Part model, mm, in its own coordinate system. A direction names the side the tool comes from. Give positions to 0.01 mm unless a question says otherwise; leave off trailing zeros. Write each loop counter-clockwise with the first axis right and the second up, starting at its lowest first coordinate (ties: lowest second). Pieces come first, ordered by that corner, then holes. Notation, with made-up numbers: (5, 84.25) - (45, 84.25) arc R29 ccw to (45, 116.25) - close; hole circle Ø6 at (56, 58). An arc over 180 degrees is marked (long way). Answer as a JSON object with one key per item and string values. Group by question number.
Autodesk Inventor part; units mm, degrees
ref_plane "YZ Plane" through (0, 0, 0) normal (1, 0, 0) x (0, 1, 0)
ref_plane "XZ Plane" through (0, 0, 0) normal (0, 1, 0) x (-1, 0, 0)
ref_plane "XY Plane" through (0, 0, 0) normal (0, 0, 1) x (1, 0, 0)
sketch "Sketch3" plane through (0, 0, 0) normal (0, 1, 0) x (-1, 0, 0)
  circle A0 centre (0, 0) radius 4.5
  circle A1 centre (0, 0) radius 2.6
  dimension "d10" = 9
  dimension "d11" = 5.2
extrude "Extrusion2" add sketch "Sketch3" along normal blind 4
sketch "Sketch4" plane through (0, 4, 0) normal (0, 1, 0) x (1, 0, 0)
  circle A0 centre (0, 0) radius 2.6
  line L0 (0, -2.6) -> (0, -1.6)
  line L1 (0, -1.6) -> (0, 2.6)
  line L2 (0, -1.6) -> (-2.0494, -1.6)
  line L3 (0, -1.6) -> (2.0494, -1.6)
  line L4 (0, 2.6) -> (0, 2.6)
  line L5 (0, 2.6) -> (0, 2.6)
  circle A1 centre (0, 0) radius 4.5
  circle A2 centre (0, 0) radius 2.6
  line L6 (0, 2.6) -> (0, 1.6)
  line L7 (0, 1.6) -> (2.0494, 1.6)
  line L8 (0, 1.6) -> (-2.0494, 1.6)
  point P0 (2.0494, 1.6)
  point P1 (-2.0494, 1.6)
  dimension "d14" = 1
  dimension "d20" = 1
extrude "Extrusion3" add sketch "Sketch4" along normal blind 6 contours L7 L1 A0 | A0 L0 L3 | L1 L8 A0 | A0 L2 L0 | A1
sketch "Sketch5" plane through (0, 10, 0) normal (0, 1, 0) x (1, 0, 0)
  circle A0 centre (0, 0) radius 4.5
extrude "Extrusion4" add sketch "Sketch5" along normal blind 1
sketch "Sketch6" plane through (2.0494, 4, 1.6) normal (0, 0, -1) x (-1, 0, 0)
  line L0 (4.0988, 6) -> (0, 6)
  line L1 (2.0494, 6) -> (2.0494, 3)
  line L2 (2.0494, 6) -> (5.0494, 6) construction
  line L3 (2.0494, 6) -> (-0.9506, 6)
  line L4 (2.0494, 6) -> (5.0494, 6) construction
  line L5 (-0.9506, 6) -> (-0.9506, 0)
  line L6 (-0.9506, 0) -> (5.0494, 0)
  line L7 (5.0494, 0) -> (5.0494, 6)
  line L8 (5.0494, 6) -> (-0.9506, 6)
  line L9 (4.6494, 6) -> (4.6494, -4)
  point P0 (2.0494, -4)
  point P1 (4.6494, 0)
  point P2 (0, 6)
  dimension "d21" = 3
  dimension "d22" = 90
  dimension "d32" = 3
  dimension "d33" = 180
  dimension "d34" = 6
  dimension "d35" = 90
  dimension "d36" = 6
  dimension "d37" = 90
extrude "Extrusion7" add sketch "Sketch6" against normal blind 46.2 contours L8 L9 L6 L5 L3 L0
sketch "Sketch8" plane through (3, 4, 3.3541) normal (1, 0, 0) x (0, 0, -1)
  line L0 (-0.3188, 6) -> (-44.4459, 6)
  line L1 (-44.4459, 6) -> (-38.4459, 6)
  line L2 (-38.4459, 6) -> (-38.4459, 0)
  line L3 (-0.3188, 0) -> (-44.4459, 0)
  line L4 (0, 6) -> (0, 0)
  line L5 (0, 6) -> (-44.4459, 6)
  line L6 (-44.4459, 0) -> (-44.4459, 6)
  line L7 (0, 0) -> (-44.4459, 0)
  point P0 (3.3541, -4)
  dimension "d40" = 6
extrude "Extrusion8" add sketch "Sketch8" against normal blind 35.56 contours L2 L3 L6 L0
sketch "Sketch10" plane through (-32.56, 4, 3.3541) normal (-1, 0, 0) x (0, 0, 1)
  line L0 (0.3188, 6) -> (38.4459, 6)
  line L1 (38.4459, 6) -> (38.4459, 13)
  line L2 (38.4459, 13) -> (31.4459, 13)
  line L3 (31.4459, 13) -> (31.4459, -7)
  line L4 (31.4459, -7) -> (51.4357, -7)
  line L5 (51.4357, -7) -> (51.4357, 13)
  line L6 (51.4357, 13) -> (38.4459, 13)
  point P0 (-3.3541, -4)
  dimension "d49" = 7
  dimension "d50" = 7
  dimension "d51" = 90
  dimension "d52" = 20
  dimension "d53" = 90
  dimension "d54" = 19.9898
  dimension "d55" = 90
  dimension "d56" = 90
extrude "Extrusion10" add sketch "Sketch10" along normal blind 3
properties part number "socket2"
1) Mould opens along X. For faces 1 (the flat face through (-34, -3, 45)), 2 (the cylindrical face through (4.037, 5.423, 1.988)), 3 (the cylindrical face through (-2.463, 4.93, 0.832)) say: pulls with the +X half, pulls with the -X half, needs draft (parallel to the pull), parting line crosses it, or undercut.
2) Drop flat-ended pins along their axis: P1, Ø0.9, axis at x = -34.5, y = 4, coming from the -Z side; P2, Ø1.8, axis at x = -9, y = 7, coming from the +Z side; P3, Ø1.8, axis at y = 8, z = 17, coming from the -X side; P4, Ø3, axis at x = -6.5, y = 1, coming from the -Z side. Give the stop position or say it passes through.
3) Which spindle directions (+Z, -Z, +X, -X, +Y, -Y) get a long thin tool onto all of the face, cutting with end or side? Do faces 4 (the flat face through (-2.6, 7, 22)), 5 (the flat face through (0, 7, -1.6)), 6 (the flat face through (-34, 7, 34.8)), 7 (the flat face through (-32.56, 7, 49)), 8 (the flat face through (-15, 7, 47.8)). Say none if no direction does.
4) Band-saw the part on A-A (y = 1). List the corners of the cut face in (x, z), plus the area to 3 significant figures.
5) Probe line 1 (Z direction, x = 0, y = 7); line 2 (X direction, y = 7.25, z = 0); line 3 (X direction, y = 14.25, z = 48). List the from-to ranges inside material, lowest first.
6) Band-saw the part on D-D (x = -21). List the corners of the cut face in (y, z).
7) Band-saw the part on B-B (y = 6.75). List the corners of the cut face in (x, z).
8) Band-saw the part on C-C (z = 44). List the corners of the cut face in (x, y).
Verdict:
{
 "1": {"face 1": "needs draft", "face 2": "parting line crosses it", "face 3": "undercut"},
 "2": {"P1": "z = 34.8", "P2": "z = 47.8", "P3": "x = -2.6", "P4": "through"},
 "3": {"face 4": "+Y, -Y", "face 5": "-Y", "face 6": "-Z, -X, +Y, -Y", "face 7": "none", "face 8": "+Z, +X, +Y, -Y"},
 "4": {"outline": "(-35.56, 34.8) - (-32.56, 34.8) - (-32.56, 54.79) - (-35.56, 54.79) - close; circle Ø9 at (0, 0); hole circle Ø5.2 at (0, 0)", "area": "102 mm2"},
 "5": {"line 1": "-4.5 to -1.6, 1.6 to 47.8", "line 2": "-4.5 to -2.6, 2.6 to 4.5", "line 3": "-35.56 to -32.56"},
 "6": {"outline": "(4, 41.8) - (10, 41.8) - (10, 47.8) - (4, 47.8) - close"},
 "7": {"outline": "(-35.56, 34.8) - (-32.56, 34.8) - (-32.56, 41.8) - (-2.6, 41.8) - (-2.6, 3.67) arc R4.5 ccw (long way) to (3, 3.35) - (3, 47.8) - (-32.56, 47.8) - (-32.56, 54.79) - (-35.56, 54.79) - close; hole (-2.05, -1.6) - (2.05, -1.6) arc R2.6 ccw to (2.05, 1.6) - (-2.05, 1.6) arc R2.6 ccw to start"},
 "8": {"outline": "(-35.56, -3) - (-32.56, -3) - (-32.56, 4) - (3, 4) - (3, 10) - (-32.56, 10) - (-32.56, 17) - (-35.56, 17) - close"}
}
